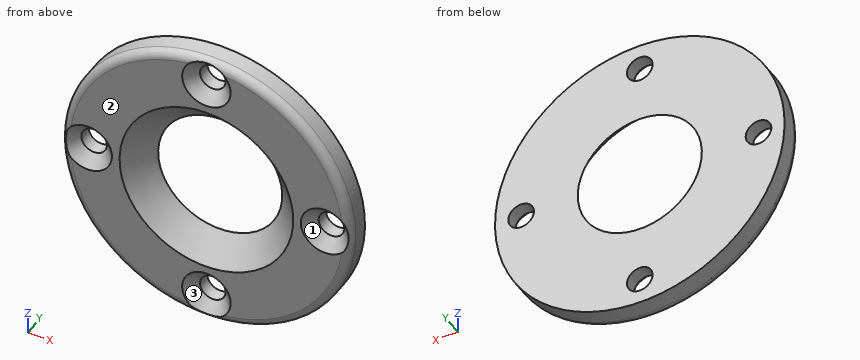
```python
from build123d import *

# Parameters (mm, degrees)
SKETCH1_R                    = 17.5
SKETCH1_R_2                  = 7.5
BOSS_EXTRUDE1_DEPTH          = 3
SKETCH3_R                    = 1.55
CUT_EXTRUDE1_DEPTH           = 5
CHAMFER6_SIZE                = 1.38
CIRPATTERN2_COUNT            = 4
CHAMFER6_OF_CIRPATTERN2_SIZE = 1.38
CHAMFER7_SIZE                = 3
FILLET1_R                    = 1


# Some blends are built 0.0001 mm under size
with BuildPart() as part:
    # Sketch1 → Boss-Extrude1 (new body)
    with BuildSketch(Plane(origin=(0, 0, 0), x_dir=(1, 0, 0), z_dir=(0, 1, 0))):
        with Locations(Location((0, 0, 0), (0, 0, 270))):
            Circle(SKETCH1_R)
        with Locations(Location((0, 0, 0), (0, 0, 270))):
            Circle(SKETCH1_R_2, mode=Mode.SUBTRACT)
    extrude(amount=BOSS_EXTRUDE1_DEPTH)

    # Sketch3 → Cut-Extrude1 (cut)
    with BuildSketch(Plane.XZ):
        with Locations(Location((0, 14.35, 0), (0, 0, 270))):
            Circle(SKETCH3_R)
    cut_extrude1 = extrude(amount=-CUT_EXTRUDE1_DEPTH, mode=Mode.SUBTRACT)

    # Chamfer6
    chamfer6_edges = [part.edges().sort_by_distance(p)[0] for p in [
        (0, 0, 15.9),
    ]]
    chamfer(chamfer6_edges, length=CHAMFER6_SIZE)

    # CirPattern2: Cut-Extrude1 ×4 about axis
    cirpattern2_axis = Axis((0, 0, 0), (0, 1, 0))
    for i in range(1, CIRPATTERN2_COUNT):
        add(cut_extrude1.rotate(cirpattern2_axis, i * 360 / CIRPATTERN2_COUNT), mode=Mode.SUBTRACT)

    # Chamfer6 of CirPattern2
    chamfer6_of_cirpattern2_edges = [part.edges().sort_by_distance(p)[0] for p in [
        (15.9, 0, 0),
        (0, 0, -15.9),
        (-15.9, 0, 0),
    ]]
    chamfer(chamfer6_of_cirpattern2_edges, length=CHAMFER6_OF_CIRPATTERN2_SIZE)

    # Chamfer7
    chamfer7_edges = [part.edges().sort_by_distance(p)[0] for p in [
        (0, 0, -7.5),
    ]]
    chamfer(chamfer7_edges, length=CHAMFER7_SIZE - 0.0001)  # a hair under: the kernel refuses the full size

    # Fillet1
    # the kernel refuses this fillet: 1 mm, written as the material it takes off along each edge
    with BuildSketch(Plane(origin=(0, 0, 0), x_dir=(0, 0, 1), z_dir=(-1, 0, 0))) as fillet1_piece_1:
        with BuildLine():
            CenterArc((17.5 - FILLET1_R, FILLET1_R), FILLET1_R, 270, 90)
            Line((17.5, FILLET1_R), (17.5, 0))
            Line((17.5, 0), (17.5 - FILLET1_R, 0))
        make_face()
    revolve(axis=Axis((0, 0, 0), (0, 1, 0)), mode=Mode.SUBTRACT)


solid = part.part
```
Model file for the job. Use its own axes, mm. Face numbers are marked on the shaded views. Give positions to 0.01 mm unless a question says otherwise; leave off trailing zeros. Write each loop counter-clockwise with the first axis right and the second up, starting at its lowest first coordinate (ties: lowest second). Pieces come first, ordered by that corner, then holes. Notation, with made-up numbers: M 47.5,79.25 L 95.5,79.25 A23 ccw 95.5,107.25 Z; hole C -19.75,-13 d10. An arc over 180 degrees is marked long. Use a Markdown table: item, result.
1) Pull direction X, two halves, no side cores. Call the marked faces 1, 2 and 3: +X half, -X half, draft (parallel to the pull), parting line (faces both ways), or undercut.
Responses:
| item | result |
|---|---|
| face 1 | undercut |
| face 2 | draft |
| face 3 | undercut |
2) Cut at A-A (z = 0). Give the number of separate pieces and of enclosed holes in the cut face, and give its area (3 significant figures).
Responses:
| item | result |
|---|---|
| separate pieces | 4 |
| enclosed holes | 0 |
| area | 28.3 mm2 |
3) Pin check, flat tips, straight feed: pin 1 (3 mm diameter, centred on x = -14.35, z = 0, fed in from -Y); pin 2 (1 mm diameter, centred on y = 0.5, z = 2, fed in from +X). Stop position of each tip, or through.
Responses:
| item | result |
|---|---|
| pin 1 | passes through |
| pin 2 | stops at x = 17.41 |
4) Cut at B-B (y = 2.45). List the corners of the cut face in (x, z).
Responses:
| item | result |
|---|---|
| outline | C 0,0 d35; hole C -14.35,0 d3.1; hole C 0,0 d16.1; hole C 0,-14.35 d3.1; hole C 0,14.35 d3.1; hole C 14.35,0 d3.1 |
5) Drill centre lines: line 1 (X direction, y = 1.8, z = -14.5); line 2 (Z direction, x = 14.35, y = 2.6); line 3 (X direction, y = 2.8, z = -15). Where is each one in solid material? Low to high. Write a range as from..to.
Responses:
| item | result |
|---|---|
| line 1 | x = -9.8..-1.54, 1.54..9.8 |
| line 2 | z = -10.02..-1.55, 1.55..10.02 |
| line 3 | x = -9.01..-1.41, 1.41..9.01 |
